```python
from build123d import *

# Parameters (mm, degrees)
F0_R         = 1.25
F1_DEPTH     = 2.5
F2_W         = 40
F2_H         = 18
F3_DEPTH     = 35
F5_DEPTH     = 40.001
F7_DEPTH     = 40
F9_DEPTH     = 10
F10_T1_DEPTH = 40
F10_T3_DEPTH = 65
F10_T5_DEPTH = 48.1285235511


# Not quite as in the source:
# - a fillet or chamfer that OpenCascade refuses, or shapes differently, is made with other operations: its cross-section is extruded or revolved along the edge and cut away or added


with BuildPart() as f1:
    # F0 (on Top) → F1 (new body)
    with BuildSketch(Plane.XY):
        with Locations((-9.5, 0)):
            Circle(F0_R)
    extrude(amount=F1_DEPTH)



with BuildPart() as f1b:
    # F0 (on Top) → F1, piece 2 (new body)
    with BuildSketch(Plane.XY):
        with Locations((9.5, 0)):
            Circle(F0_R)
    extrude(amount=F1_DEPTH)


with BuildPart() as f1_1:
    add(f1.part)

    add(f1b.part)  # F3 merges F1b
    # F2 (on Top) → F3 (join)
    with BuildSketch(Plane.XY):
        with Locations((0, -6)):
            Rectangle(F2_W, F2_H)
    extrude(amount=-F3_DEPTH)

    # F4 (on face) → F5 (cut, through all)
    with BuildSketch(Plane(origin=(-20, 0, 0), x_dir=(0, -1, 0), z_dir=(-1, 0, 0))):
        with BuildLine():
            Line((-3, -35), (11, -35))
            ThreePointArc((11, -35), (7.459306232, -17.9377326694), (-3, -4))
            Line((-3, -4), (-3, -35))
        make_face()
    extrude(amount=-F5_DEPTH, mode=Mode.SUBTRACT)

    # F6 (on face) → F7 (join)
    with BuildSketch(Plane(origin=(-20, 0, 0), x_dir=(0, -1, 0), z_dir=(-1, 0, 0))):
        with BuildLine():
            Line((-3, 10), (2, 10))
            ThreePointArc((2, 10), (8.5, 14.1331594945), (15, 10))
            ThreePointArc((15, 10), (18.881651405, 5), (15, 0))
            Line((15, 0), (15, -7.1779969148))
            Line((15, -7.1779969148), (20.2195104212, 0))
            Line((20.2195104212, 0), (20.2195104212, 15))
            Line((20.2195104212, 15), (-3, 15))
            Line((-3, 15), (-3, 10))
        make_face()
    extrude(amount=-F7_DEPTH)

    # F8 (on face) → F9 (cut)
    with BuildSketch(Plane(origin=(0, 3, 0), x_dir=(-1, 0, 0), z_dir=(0, 1, 0))):
        Polygon((9.1120566488, 3.2700138061), (11, 0), (11, 3.2700138061), align=None)
        Polygon((-9.8879433512, 3.2700138061), (-8, 0), (-8, 3.2700138061), align=None)
    extrude(amount=-F9_DEPTH, mode=Mode.SUBTRACT)

    # F10: fillet of radius 5 on 5 edges, made by hand

    # F10_s2 → F10_t1 (join)
    with BuildSketch(Plane.YZ.offset(-20)):
        with BuildLine():
            ThreePointArc((-15, -8.803701625), (-15.245026694, -7.257665125), (-15.9560915438, -5.8631567099))
            Line((-15.9560915438, -5.8631567099), (-15, -7.1779969148))
            Line((-15, -7.1779969148), (-15, -8.803701625))
        make_face()
    extrude(amount=F10_T1_DEPTH)

    # F10_s4 → F10_t3 (cut)
    with BuildSketch(Plane.YZ.offset(-32.5)):
        with BuildLine():
            ThreePointArc((-20.2195104212, 10), (-18.7550443271, 13.5355339059), (-15.2195104212, 15))
            Line((-15.2195104212, 15), (-20.2195104212, 15))
            Line((-20.2195104212, 15), (-20.2195104212, 10))
        make_face()
        with BuildLine():
            ThreePointArc((-2, 15), (1.5355339059, 13.5355339059), (3, 10))
            Line((3, 10), (3, 15))
            Line((3, 15), (-2, 15))
        make_face()
        with BuildLine():
            ThreePointArc((3, 15), (1.5355339059, 11.4644660941), (-2, 10))
            Line((-2, 10), (3, 10))
            Line((3, 10), (3, 15))
        make_face()
    extrude(amount=F10_T3_DEPTH, mode=Mode.SUBTRACT)

    # F10_s6 → F10_t5 (cut)
    with BuildSketch(Plane.YZ.offset(-24.0642617755)):
        with BuildLine():
            ThreePointArc((-19.2634188773, -1.314840205), (-19.9744837271, 0.0796682101), (-20.2195104212, 1.6257047102))
            Line((-20.2195104212, 1.6257047102), (-20.2195104212, 0))
            Line((-20.2195104212, 0), (-19.2634188773, -1.314840205))
        make_face()
    extrude(amount=F10_T5_DEPTH, mode=Mode.SUBTRACT)


solid = f1_1.part
```
Geometry check sheet. Reference: the model listing, model coordinates, mm. A direction names the side the tool comes from. Give positions to 0.01 mm unless a question says otherwise; leave off trailing zeros. Write each loop counter-clockwise with the first axis right and the second up, starting at its lowest first coordinate (ties: lowest second). Pieces come first, ordered by that corner, then holes. Notation, with made-up numbers: (60, 49.25) - (97, 49.25) arc R13 ccw to (97, 67.25) - close; hole circle Ø4 at (47.25, 60). An arc over 180 degrees is marked (long way). Use a Markdown table: item, result.
Q1. Section check B-B, the plane x = -12. Enter the section's corners in (y, z).
Computed:
| item | result |
|---|---|
| outline | (-20.22, 1.63) arc R5 ccw to (-19.26, -1.31) - (-15.96, -5.86) arc R5 cw to (-15, -8.8) - (-15, -35) - (-11, -35) arc R40 cw to (3, -4) - (3, 0) - (-15, 0) arc R5.16 cw to (-15, 10) arc R7.18 cw to (-2, 10) arc R5 ccw to (2.33, 12.5) arc R5 ccw to (-2, 15) - (-15.22, 15) arc R5 ccw to (-20.22, 10) - close |
Q2. Section check C-C, the plane y = -5.5. Enter the section's corners in (x, z), then the cut area to 3 significant figures.
Computed:
| item | result |
|---|---|
| outline | (-20, -14.15) - (20, -14.15) - (20, 0) - (-20, 0) - close; (-20, 13.48) - (20, 13.48) - (20, 15) - (-20, 15) - close |
| area | 627 mm² |
Q3. Section check A-A, the plane y = -9. Enter the section's corners in (x, z), then the cut area to 3 significant figures.
Computed:
| item | result |
|---|---|
| outline | (-20, -21.9) - (20, -21.9) - (20, 0) - (-20, 0) - close; (-20, 14.12) - (20, 14.12) - (20, 15) - (-20, 15) - close |
| area | 911 mm² |
Q4. Thickness scan on L1, parallel to Z at x = 17.5, y = -4.5; L2, parallel to Z at x = 10, y = -2.5; L3, parallel to Y at x = 10.5, z = -3. Record the ranges inside material, lowest first. Write a range as [from, to].
Computed:
| item | result |
|---|---|
| L1 | z = [-12.54, 0], [12.92, 15] |
| L2 | z = [-9.74, 0], [10.89, 15] |
| L3 | y = [-18.04, 3] |
Q5. Go/stop test with flat-tipped pins: P1, Ø2, axis at x = 2, y = -1.5, coming from the -Z side; P2, Ø2, axis at x = -12, z = -18.5, coming from the -Y side; P3, Ø10, axis at y = -8, z = 6, coming from the +X side; P4, Ø4, axis at y = -9.5, z = -24.5, coming from the +X side. Record where each tip stops, or that it passes through.
Computed:
| item | result |
|---|---|
| P1 | stops at z = -9.74 |
| P2 | stops at y = -15 |
| P3 | passes through |
| P4 | stops at x = 20 |
Q6. Set-up check for faces 4 (the face through (10, 0, 2.5)), 5 (the face through (8.988, 0.017, 1.711)), 6 (the face through (-0.28, -8.386, 14.132)): record each of +Z, -Z, +X, -X, +Y, -Y from which the full face is reachable in a straight line by a thin tool's end or side.
Computed:
| item | result |
|---|---|
| face 4 | +X, -X, +Y |
| face 5 | +Y |
| face 6 | +X, -X |
Q7. Section check D-D, the plane z = -12. Enter the section's corners in (x, y), then the cut area to 3 significant figures.
Computed:
| item | result |
|---|---|
| outline | (-20, -15) - (20, -15) - (20, -4.14) - (-20, -4.14) - close |
| area | 434 mm² |
Q8. Draft check along X on faces 1 (the face through (-20, -11, -4)), 2 (the face through (-8.31, 0.38, 0.95)), 3 (the face through (-0.28, -18.88, 5.1)). Enter one of: pulls with the +X half, pulls with the -X half, needs draft (parallel to the pull), parting line crosses it, or undercut.
Computed:
| item | result |
|---|---|
| face 1 | pulls with the -X half |
| face 2 | undercut |
| face 3 | needs draft |
